Geometry check sheet. Reference: the model listing, model coordinates, mm. Coordinates: 2 decimals unless noted, no trailing zeros. Write each loop counter-clockwise with the first axis right and the second up, starting at its lowest first coordinate (ties: lowest second). Pieces come first, ordered by that corner, then holes.
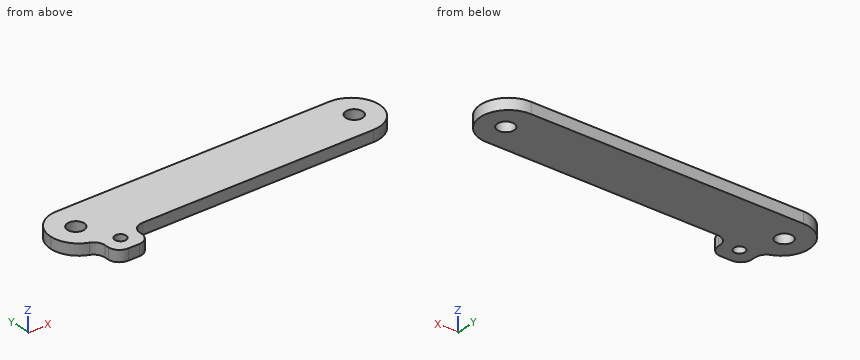
from build123d import *

# Parameters (mm, degrees)
SKETCH1_R           = 1.5
SKETCH1_R_2         = 1
BOSS_EXTRUDE1_DEPTH = 2
FILLET2_R           = 5
FILLET3_R           = 2


with BuildPart() as part:
    # Sketch1 → Boss-Extrude1 (new body)
    with BuildSketch(Plane.XY):
        Polygon((0, 0), (0, 10), (59, 10), (59, 0), (10.458327832, 0), (10.458327832, -4.344154509), (4.458327832, -4.344154509), (4.458327832, 0), align=None)
        with Locations((4.5, 5)):
            Circle(SKETCH1_R, mode=Mode.SUBTRACT)
        with Locations((54.5, 5)):
            Circle(SKETCH1_R, mode=Mode.SUBTRACT)
        with Locations((7.458327832, -1.344154509)):
            Circle(SKETCH1_R_2, mode=Mode.SUBTRACT)
    extrude(amount=BOSS_EXTRUDE1_DEPTH)

    # Fillet2
    # the kernel refuses this fillet: 5 mm, written as the material it takes off along each edge
    with BuildSketch(Plane(origin=(59, 0, -12.5), x_dir=(0, 1, 0), z_dir=(0, 0, 1)), Plane(origin=(59, 10, -12.5), x_dir=(-1, 0, 0), z_dir=(0, 0, 1)), Plane(origin=(0, 10, -12.5), x_dir=(0, -1, 0), z_dir=(0, 0, 1))) as fillet2_piece_1:
        with BuildLine():
            CenterArc((FILLET2_R, FILLET2_R), FILLET2_R, 180, 90)
            Line((0, FILLET2_R), (-FILLET2_R * 0.02, FILLET2_R))
            Line((-FILLET2_R * 0.02, FILLET2_R), (-FILLET2_R * 0.02, -FILLET2_R * 0.02))
            Line((-FILLET2_R * 0.02, -FILLET2_R * 0.02), (FILLET2_R, -FILLET2_R * 0.02))
            Line((FILLET2_R, -FILLET2_R * 0.02), (FILLET2_R, 0))
        make_face()
    extrude(amount=27, mode=Mode.SUBTRACT)
    with BuildSketch(Plane(origin=(0, 0, -12.426431322), x_dir=(0, 1, 0), z_dir=(0, 0, 1))) as fillet2_piece_2:
        with BuildLine():
            CenterArc((4.970572529, -5), FILLET2_R, 90, 83.780688145)
            Line((0, -4.458327832), (-0.099411451, -4.447494389))
            ThreePointArc((-0.099411451, -4.447494389), (-0.1, -2.229163916), (-0.1, 0))
            Line((-0.1, 0), (0, 0.1))
            Line((0, 0.1), (4.970572529, 0.1))
            Line((4.970572529, 0.1), (4.970572529, 0))
        make_face()
    extrude(amount=26.852862643, mode=Mode.SUBTRACT)

    # Fillet3
    fillet3_edges = [part.edges().sort_by_distance(p)[0] for p in [
        (10.458327832, 0, 1),
        (10.458327832, -4.344154509, 1),
        (4.458327832, -4.344154509, 1),
        (4.458327832, 0, 1),
    ]]
    fillet(fillet3_edges, radius=FILLET3_R)


solid = part.part
1. Sectioned sample at D-D, the plane y = 9. Record the boundary of the cut face in (x, z).
Computed values:
outline: (2, 0) - (57, 0) - (57, 2) - (2, 2) - close
2. Sectioned sample at B-B, the plane z = 1.7. Give the number of separate pieces and of enclosed holes in the cut face, and give its area (3 significant figures).
Computed values:
separate pieces: 1
enclosed holes: 3
area: 577 mm2
3. Sectioned sample at A-A, the plane y = 4.25. Record the boundary of the cut face in (x, z).
Computed values:
outline: (0.05, 0) - (3.2, 0) - (3.2, 2) - (0.05, 2) - close; (5.8, 0) - (53.2, 0) - (53.2, 2) - (5.8, 2) - close; (55.8, 0) - (58.94, 0) - (58.94, 2) - (55.8, 2) - close
4. Thickness scan on line 1 along X through (y, z) = (6, 1.55); line 2 along X through (y, z) = (4.5, 1.7); line 3 along Y through (x, z) = (17, 0.3). Record the ranges inside material, lowest first.
Computed values:
line 1: x = 0.1 to 3.38, 5.62 to 53.38, 55.62 to 58.9
line 2: x = 0.02 to 3.09, 5.91 to 53.09, 55.91 to 58.97
line 3: y = 0 to 10
5. Sectioned sample at C-C, the plane x = 54.5. Record the boundary of the cut face in (y, z), and give its area (3 significant figures).
Computed values:
outline: (0.03, 0) - (3.5, 0) - (3.5, 2) - (0.03, 2) - close; (6.5, 0) - (9.97, 0) - (9.97, 2) - (6.5, 2) - close
area: 13.9 mm2
6. Gauge pin test, flat ends, axial feed: pin 1 Ø2 at (x, y) = (29.5, 8) entering from -Z; pin 2 Ø1 at (y, z) = (3, 1) entering from -X; pin 3 Ø1 at (y, z) = (7.5, 1) entering from +X. Record the tip position at first contact, or that the pin passes through.
Computed values:
pin 1: stops at z = 0
pin 2: stops at x = 0.22
pin 3: stops at x = 58.58
